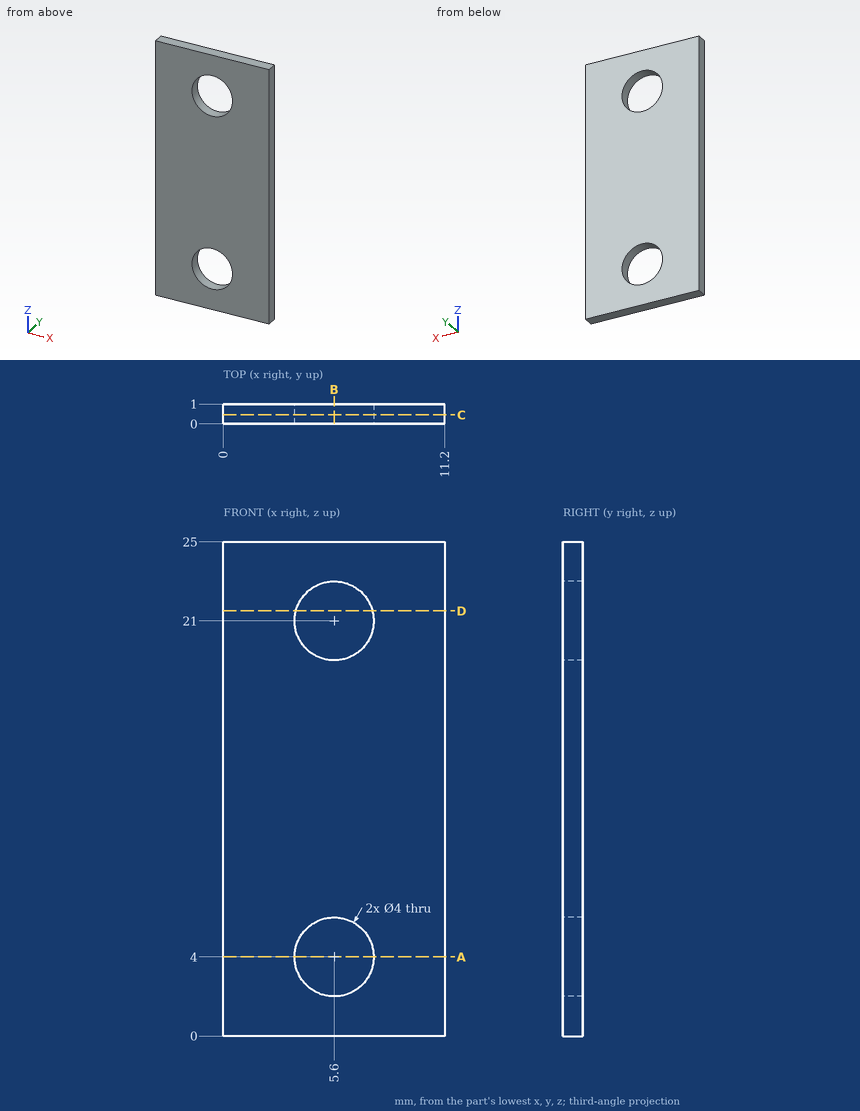
Can you work these out from the drawing? Everything is in mm from the part's minimum corner. Give positions to 0.01 mm unless a question says otherwise; leave off trailing zeros. Loops run counter-clockwise (first coordinate to the right, second up) from the corner with the lowest first, then second, coordinate; pieces in that order, holes last. Notation, with made-up numbers: (-3.5, 77) -> (15.5, 77) arc R22 cw to (15.5, 102) -> close; hole circle Ø4 at (71.5, 48.25). An arc over 180 degrees is marked (long way). Put each result on its own line as item: value.
(1) Imagine slicing it at D-D on z = 21.5. Write out the boundary of the cut face in (x, y), plus the area to 3 significant figures.
Computed:
outline: (0, 0) -> (3.66, 0) -> (3.66, 1) -> (0, 1) -> close; (7.54, 0) -> (11.2, 0) -> (11.2, 1) -> (7.54, 1) -> close
area: 7.33 mm^2
(2) Please list where these lines run through material, in increasing order: probe 1 along Z at (x, y) = (5.6, 0.6); probe 2 along Z at (x, y) = (4, 0.55); probe 3 along X at (y, z) = (0.2, 20.5). Write a range as [from, to].
Computed:
probe 1: [0, 2], [6, 19], [23, 25]
probe 2: [0, 2.8], [5.2, 19.8], [22.2, 25]
probe 3: [0, 3.66], [7.54, 11.2]
(3) Imagine slicing it at B-B on x = 5.6. Write out the boundary of the cut face in (y, z), plus the area to 3 significant figures.
Computed:
outline: (0, 0) -> (1, 0) -> (1, 2) -> (0, 2) -> close; (0, 6) -> (1, 6) -> (1, 19) -> (0, 19) -> close; (0, 23) -> (1, 23) -> (1, 25) -> (0, 25) -> close
area: 17.0 mm^2
(4) Imagine slicing it at A-A on z = 4. Write out the boundary of the cut face in (x, y), plus the area to 3 significant figures.
Computed:
outline: (0, 0) -> (3.6, 0) -> (3.6, 1) -> (0, 1) -> close; (7.6, 0) -> (11.2, 0) -> (11.2, 1) -> (7.6, 1) -> close
area: 7.20 mm^2
(5) Imagine slicing it at C-C on y = 0.45. Write out the boundary of the cut face in (x, z), plus the area to 3 significant figures.
Computed:
outline: (0, 0) -> (11.2, 0) -> (11.2, 25) -> (0, 25) -> close; hole circle Ø4 at (5.6, 4); hole circle Ø4 at (5.6, 21)
area: 255 mm^2
